CAD build for the part. Positions are in the model's coordinates, mm. Give positions to 0.01 mm unless a question says otherwise; leave off trailing zeros. Order: outer loops, then holes, each group sorted by start corner. A loop starts at its lowest first (then second) coordinate and runs counter-clockwise, first axis right, second up. Notation, with made-up numbers: (10, 15) -> (14, 15) arc R34 ccw to (14, 48) -> close; hole circle Ø4 at (55, -27.75). An arc over 180 degrees is marked (long way). Use one line per item in the form item = value. Start each with the question number.
1) Cut at C-C, the plane y = 442.5. Give the cut face in (x, z), and give its area (3 significant figures).
2) Cut at A-A, the plane z = 0. Give the cut face in (x, y).
3) Drop flat-ended pins along their axis: P1, Ø3, axis at y = 352, z = 14, coming from the -X side; P2, Ø3, axis at y = 658.5, z = -40, coming from the -X side; P3, Ø3, axis at x = 16, y = 339.5, coming from the +Z side. Give the stop position or say it passes through.
4) Cut at B-B, the plane x = 0. Give the cut face in (y, z), and give its area (3 significant figures).
5) Probe line 1 (X direction, y = 291.5, z = 0); line 2 (Z direction, x = 12, y = 171). List the from-to ranges inside material, lowest first.
6) Mould opens along X. For faces 1 (the face through (-40.434, 413.233, 31.004)), 2 (the face through (11, 0, 49)), 3 (the face through (45.8, 413.23, 18.99)) say: pulls with the +X half, pulls with the -X half, needs draft (parallel to the pull), parting line crosses it, or undercut.
from build123d import *

# Parameters (mm, degrees)
SKETCH2_R           = 50.9524
SKETCH2_R_2         = 49.5808
BOSS_EXTRUDE1_DEPTH = 838.2
SKETCH3_W           = 2.9972
SKETCH3_H           = 302.26
CUT_EXTRUDE1_DEPTH  = 51.9524
CIRPATTERN2_COUNT   = 3


with BuildPart() as part:
    # Sketch2 → Boss-Extrude1 (new body)
    with BuildSketch(Plane(origin=(0, 0, 0), x_dir=(1, 0, 0), z_dir=(0, 1, 0))):
        Circle(SKETCH2_R)
        Circle(SKETCH2_R_2, mode=Mode.SUBTRACT)
    extrude(amount=BOSS_EXTRUDE1_DEPTH)

    # Sketch3 → Cut-Extrude1 (cut, through all)
    with BuildSketch(Plane.XY):
        with Locations((-11.027101343, 162.4838)):
            Rectangle(SKETCH3_W, SKETCH3_H)
    cut_extrude1 = extrude(amount=-CUT_EXTRUDE1_DEPTH, mode=Mode.SUBTRACT)

    # CirPattern2: Cut-Extrude1 ×3 about axis
    cirpattern2_axis = Axis((0, 0, 0), (0, 1, 0))
    for i in range(1, CIRPATTERN2_COUNT):
        add(cut_extrude1.rotate(cirpattern2_axis, i * 360 / CIRPATTERN2_COUNT), mode=Mode.SUBTRACT)


solid = part.part
Result:
q1.outline = circle Ø101.9 at (0, 0); hole circle Ø99.16 at (0, 0)
q1.area = 433 mm²
q2.outline = (-50.95, 0) -> (-49.58, 0) -> (-49.58, 838.2) -> (-50.95, 838.2) -> close; (49.58, 0) -> (50.95, 0) -> (50.95, 838.2) -> (49.58, 838.2) -> close
q3.P1 = -49.4
q3.P2 = -33.38
q3.P3 = 48.85
q4.outline = (0, -50.95) -> (838.2, -50.95) -> (838.2, -49.58) -> (0, -49.58) -> close; (0, 49.58) -> (838.2, 49.58) -> (838.2, 50.95) -> (0, 50.95) -> close
q4.area = 2,300 mm²
q5.line_1 = -50.95 to -49.58, 49.58 to 50.95
q5.line_2 = -49.52 to -48.11, 48.11 to 49.52
q6.face_1 = parting line crosses it
q6.face_2 = needs draft
q6.face_3 = undercut
